```python
from build123d import *
from build123d.topology import SkipClean

# Parameters (mm, degrees)
CROQUIS1_R                          = 15
CROQUIS1_R_2                        = 10.5
SALIENTE_EXTRUIR1_DEPTH             = 4
CROQUIS2_R                          = 1.875
CORTAR_EXTRUIR1_DEPTH               = 8
SALIENTE_EXTRUIR2_REACH             = 35.779
SALIENTE_EXTRUIR2_END_RADIUS        = 15
CROQUIS2_4_R                        = 1.875
SALIENTE_EXTRUIR2_DIRECTION_2_DEPTH = 2
REVOLUCI_N1_ANGLE                   = 20
REVOLUCI_N1_OTHER_WAY_ANGLE         = 20
CORTAR_EXTRUIR6_DEPTH               = 35.481879299
CORTAR_EXTRUIR6_DEPTH_BACK          = 3
CROQUIS4_3_R                        = 1.875
CORTAR_EXTRUIR7_DEPTH               = 35.481879299
CORTAR_EXTRUIR8_START               = -8
CORTAR_EXTRUIR8_DEPTH               = 8
REDONDEO3_R                         = 1
SALIENTE_EXTRUIR3_START             = 5
SALIENTE_EXTRUIR3_DEPTH             = 5
CORTAR_EXTRUIR9_DEPTH               = 1.75
CORTAR_EXTRUIR9_DEPTH_BACK          = 0.5
SALIENTE_EXTRUIR4_OUTLINE_R         = 1.875
SALIENTE_EXTRUIR4_DEPTH             = 2.75
CORTAR_EXTRUIR10_DEPTH              = 3


# Read off the part's stored shape, not the designer's step: Cortar-Extruir8, Saliente-Extruir4
with BuildPart() as part:
    # Croquis1 → Saliente-Extruir1 (new, symmetric)
    with BuildSketch(Plane(origin=(0, 0, 0), x_dir=(1, 0, 0), z_dir=(0, 1, 0))):
        with Locations(Location((0, 0, 0), (0, 0, 270))):
            Circle(CROQUIS1_R)
        with Locations(Location((0, 0, 0), (0, 0, 270))):
            Circle(CROQUIS1_R_2, mode=Mode.SUBTRACT)
    extrude(amount=SALIENTE_EXTRUIR1_DEPTH, both=True)

    # Croquis2 → Cortar-Extruir1 (cut)
    with BuildSketch(Plane(origin=(0, 0, -15), x_dir=(-1, 0, 0), z_dir=(0, 0, -1))):
        Polygon((-3.2, 0), (-1.6, -2.771281292), (1.6, -2.771281292), (3.2, 0), (1.6, 2.771281292), (-1.6, 2.771281292), align=None)
        Circle(CROQUIS2_R)
    extrude(amount=-CORTAR_EXTRUIR1_DEPTH, mode=Mode.SUBTRACT)

    # Saliente-Extruir2: up to this cylinder (the profile starts outside it)
    with SkipClean():  # the faces are left unmerged after this step: merging them gives an invalid solid
        saliente_extruir2_end = Plane(origin=(0, -1.641104, 0), z_dir=(0, -1, 0)) * Cylinder(SALIENTE_EXTRUIR2_END_RADIUS, 103.15359, mode=Mode.PRIVATE)
        # Croquis2<4> → Saliente-Extruir2 (add, up to the surface)
        with BuildSketch(Plane(origin=(0, 0, -15), x_dir=(-1, 0, 0), z_dir=(0, 0, -1)), mode=Mode.PRIVATE) as saliente_extruir2_sk1:
            Polygon((-4.618802154, 0), (-2.309401077, -4), (2.309401077, -4), (4.618802154, 0), (2.309401077, 4), (-2.309401077, 4), align=None)
            Polygon((-1.6, -2.771281292), (1.6, -2.771281292), (3.2, 0), (1.6, 2.771281292), (-1.6, 2.771281292), (-3.2, 0), align=None, mode=Mode.SUBTRACT)
        saliente_extruir2_tool1 = extrude(saliente_extruir2_sk1.sketch, amount=-SALIENTE_EXTRUIR2_REACH, mode=Mode.PRIVATE) - saliente_extruir2_end
        add(saliente_extruir2_tool1.solids().sort_by_distance((3.358272, -1.938899, -15))[0])
        add(saliente_extruir2_tool1.solids().sort_by_distance((3.358272, -1.938899, -15))[1])
        # Croquis2<4> → Saliente-Extruir2 (add, up to the surface)
        with BuildSketch(Plane(origin=(0, 0, -15), x_dir=(-1, 0, 0), z_dir=(0, 0, -1)), mode=Mode.PRIVATE) as saliente_extruir2_sk2:
            Polygon((-3.2, 0), (-1.6, -2.771281292), (1.6, -2.771281292), (3.2, 0), (1.6, 2.771281292), (-1.6, 2.771281292), align=None)
            Circle(CROQUIS2_4_R, mode=Mode.SUBTRACT)
        saliente_extruir2_tool2 = extrude(saliente_extruir2_sk2.sketch, amount=-SALIENTE_EXTRUIR2_REACH, mode=Mode.PRIVATE) - saliente_extruir2_end
        add(saliente_extruir2_tool2.solids().sort_by_distance((2.326679, -1.343309, -15))[0])
        add(saliente_extruir2_tool2.solids().sort_by_distance((2.326679, -1.343309, -15))[1])

    # Croquis2<4> → Saliente-Extruir2 direction 2 (add)
    # profile 1 of 2: a face of its own
    with BuildSketch(Plane(origin=(0, 0, -15), x_dir=(-1, 0, 0), z_dir=(0, 0, -1))):
        Polygon((-4.618802154, 0), (-2.309401077, -4), (2.309401077, -4), (4.618802154, 0), (2.309401077, 4), (-2.309401077, 4), align=None)
        Polygon((-1.6, -2.771281292), (1.6, -2.771281292), (3.2, 0), (1.6, 2.771281292), (-1.6, 2.771281292), (-3.2, 0), align=None, mode=Mode.SUBTRACT)
    # profile 2 of 2: a face of its own
    with BuildSketch(Plane(origin=(0, 0, -15), x_dir=(-1, 0, 0), z_dir=(0, 0, -1))):
        Polygon((-3.2, 0), (-1.6, -2.771281292), (1.6, -2.771281292), (3.2, 0), (1.6, 2.771281292), (-1.6, 2.771281292), align=None)
        Circle(CROQUIS2_4_R, mode=Mode.SUBTRACT)
    extrude(amount=SALIENTE_EXTRUIR2_DIRECTION_2_DEPTH)

    # Croquis3 → Revolución1 (revolve)
    with BuildSketch(Plane(origin=(0, 0, 0), x_dir=(0, 0, -1), z_dir=(1, 0, 0))):
        Polygon((-30, 4), (-14, 4), (-14, -4), (-30, -4), (-30, -2.5), (-15, -2.5), (-15, 2.5), (-30, 2.5), align=None)
    revolve(axis=Axis((0, 4, 0), (0, -1, 0)), revolution_arc=REVOLUCI_N1_ANGLE)

    # Croquis3 → Revolución1 other way (revolve)
    with BuildSketch(Plane(origin=(0, 0, 0), x_dir=(0, 0, -1), z_dir=(1, 0, 0))):
        Polygon((-30, 4), (-14, 4), (-14, -4), (-30, -4), (-30, -2.5), (-15, -2.5), (-15, 2.5), (-30, 2.5), align=None)
    revolve(axis=Axis((0, 4, 0), (0, 1, 0)), revolution_arc=REVOLUCI_N1_OTHER_WAY_ANGLE)

    # Croquis4 → Cortar-Extruir6 (cut, two sides: drawn at the far end of the back side and taken through both)
    with BuildSketch(Plane.XZ.offset(4).offset(-CORTAR_EXTRUIR6_DEPTH_BACK)):
        with BuildLine():
            ThreePointArc((8.584705597, 23.586284782), (4.358569265, 24.7186746), (1.2e-08, 25.1))
            ThreePointArc((1.2e-08, 25.1), (-3.1, 22.000000006), (0, 18.9))
            ThreePointArc((0, 18.9), (3.281950558, 18.612866532), (6.464180709, 17.760190533))
            Line((6.464180709, 17.760190533), (8.584705597, 23.586284782))
        make_face()
    extrude(amount=CORTAR_EXTRUIR6_DEPTH + CORTAR_EXTRUIR6_DEPTH_BACK, mode=Mode.SUBTRACT)

    # Croquis4<3> → Cortar-Extruir7 (cut, through all)
    with BuildSketch(Plane.XZ.offset(4)):
        with Locations(Location((0, 22, 0), (0, 0, 270))):
            Circle(CROQUIS4_3_R)
    extrude(amount=-CORTAR_EXTRUIR7_DEPTH, mode=Mode.SUBTRACT)

    # Cortar-Extruir8 outline → Cortar-Extruir8 (cut)
    with BuildSketch(Plane.XZ.offset(4).offset(CORTAR_EXTRUIR8_START)):
        with BuildLine():
            ThreePointArc((-7.184552477, 19.7393957), (-6.262942497, 26.739718497), (1e-09, 30))
            ThreePointArc((1e-09, 30), (-5.20944533, 29.544232591), (-10.2606043, 28.190778624))
            Line((-10.2606043, 28.190778624), (-7.184552477, 19.7393957))
        make_face()
        with BuildLine():
            Line((7.184552477, 19.7393957), (8.584705598, 23.586284782))
            Line((8.584705598, 23.586284782), (10.2606043, 28.190778624))
            ThreePointArc((10.2606043, 28.190778624), (5.209445331, 29.54423259), (1e-09, 30))
            ThreePointArc((1e-09, 30), (6.262942498, 26.739718496), (7.184552477, 19.7393957))
        make_face()
    extrude(amount=CORTAR_EXTRUIR8_DEPTH, mode=Mode.SUBTRACT)

    # Redondeo3
    redondeo3_edges = [part.edges().sort_by_distance(p)[0] for p in [
        (6.464180709, -3.25, 17.760190533),
        (7.474898271, -3.25, 23.961133025),
        (-5.13030215, 3.25, 14.095389312),
        (-5.13030215, -3.25, 14.095389312),
        (5.13030215, 3.25, 14.095389312),
        (5.13030215, -3.25, 14.095389312),
    ]]
    fillet(redondeo3_edges, radius=REDONDEO3_R)

    # Croquis9 → Saliente-Extruir3 (add)
    with BuildSketch(Plane(origin=(0, -2.5, 0), x_dir=(1, 0, 0), z_dir=(0, 1, 0)).offset(SALIENTE_EXTRUIR3_START)):
        with BuildLine():
            Line((6.112599464, -16.794229002), (5.461623706, -15.005687805))
            ThreePointArc((5.461623706, -15.005687805), (5.482238333, -14.26959198), (6.001234056, -13.747188433))
            ThreePointArc((6.001234056, -13.747188433), (0, -15), (-6.001234056, -13.747188433))
            ThreePointArc((-6.001234056, -13.747188433), (-5.482238333, -14.26959198), (-5.461623706, -15.005687805))
            Line((-5.461623706, -15.005687805), (-7.184552477, -19.7393957))
            ThreePointArc((-7.184552477, -19.7393957), (-3.08103884, -29.351717504), (6.779967306, -25.888177056))
            ThreePointArc((6.779967306, -25.888177056), (6.683772805, -24.813619231), (5.667398999, -24.451801336))
            ThreePointArc((5.667398999, -24.451801336), (2.852173422, -24.93742382), (0, -25.1))
            ThreePointArc((0, -25.1), (-3.1, -22), (0, -18.9))
            ThreePointArc((0, -18.9), (2.760553354, -18.697308501), (5.461896053, -18.0935815))
            ThreePointArc((5.461896053, -18.0935815), (6.067051121, -17.584028122), (6.112599464, -16.794229002))
        make_face()
    extrude(amount=-SALIENTE_EXTRUIR3_DEPTH)

    # Croquis10 → Cortar-Extruir9 (cut, two sides: drawn at the far end of the back side and taken through both)
    with BuildSketch(Plane(origin=(0, -0.75, 0), x_dir=(-1, 0, 0), z_dir=(0, -1, 0)).offset(-CORTAR_EXTRUIR9_DEPTH_BACK)):
        with BuildLine():
            ThreePointArc((-6.779967306, -25.888177056), (-6.668671988, -26.09396334), (-6.551132513, -26.296248074))
            ThreePointArc((-6.551132513, -26.296248074), (-3.300127057, -26.898311497), (0, -27.1))
            ThreePointArc((0, -27.1), (5.1, -22), (0, -16.9))
            ThreePointArc((0, -16.9), (-1.942951583, -16.787940289), (-3.860136706, -16.453247236))
            ThreePointArc((-3.860136706, -16.453247236), (-4.828629021, -16.195503752), (-5.780140422, -15.880805291))
            Line((-5.780140422, -15.880805291), (-6.112599464, -16.794229002))
            ThreePointArc((-6.112599464, -16.794229002), (-6.067051121, -17.584028122), (-5.461896053, -18.0935815))
            ThreePointArc((-5.461896053, -18.0935815), (-2.760553354, -18.697308501), (0, -18.9))
            ThreePointArc((0, -18.9), (3.1, -22), (0, -25.1))
            ThreePointArc((0, -25.1), (-2.852173422, -24.93742382), (-5.667398999, -24.451801336))
            ThreePointArc((-5.667398999, -24.451801336), (-6.683772805, -24.813619231), (-6.779967306, -25.888177056))
        make_face()
    extrude(amount=CORTAR_EXTRUIR9_DEPTH + CORTAR_EXTRUIR9_DEPTH_BACK, mode=Mode.SUBTRACT)

    # Saliente-Extruir4 outline → Saliente-Extruir4 (add)
    with BuildSketch(Plane.XZ.offset(-2.5)):
        with BuildLine():
            ThreePointArc((5.461896053, 18.0935815), (6.067051121, 17.584028122), (6.112599464, 16.794229002))
            Line((6.112599464, 16.794229002), (7.184552477, 19.7393957))
            ThreePointArc((7.184552477, 19.7393957), (7.629143545, 22.856350834), (6.779967306, 25.888177056))
            ThreePointArc((6.779967306, 25.888177056), (6.683772805, 24.813619231), (5.667398999, 24.451801336))
            ThreePointArc((5.667398999, 24.451801336), (2.852173422, 24.93742382), (0, 25.1))
            ThreePointArc((0, 25.1), (-3.1, 22), (0, 18.9))
            ThreePointArc((0, 18.9), (2.760553354, 18.697308501), (5.461896053, 18.0935815))
        make_face()
        with Locations((0, 22)):
            Circle(SALIENTE_EXTRUIR4_OUTLINE_R, mode=Mode.SUBTRACT)
    extrude(amount=SALIENTE_EXTRUIR4_DEPTH)

    # Croquis12 → Cortar-Extruir10 (cut)
    with BuildSketch(Plane.XZ.offset(0.25)):
        Polygon((-2.771281292, 23.6), (-2.771281292, 20.4), (0, 18.8), (2.771281292, 20.4), (2.771281292, 23.6), (0, 25.2), align=None)
    extrude(amount=-CORTAR_EXTRUIR10_DEPTH, mode=Mode.SUBTRACT)


solid = part.part
```
Verification items for the finished model (mm, model axes). A direction names the side the tool comes from. Give positions to 0.01 mm unless a question says otherwise; leave off trailing zeros. Order: outer loops, then holes, each group sorted by start corner. A loop starts at its lowest first (then second) coordinate and runs counter-clockwise, first axis right, second up. Notation, with made-up numbers: (76, 63) -> (111, 63) arc R31 ccw to (111, 99) -> close; hole circle Ø9 at (-23, 69.25). An arc over 180 degrees is marked (long way). Use a Markdown table: item, result.
1) Section check C-C, the plane y = 0.5. Record the boundary of the cut face in (x, z), then the cut area to 3 significant figures.
Results:
| item | result |
|---|---|
| outline | (-7.18, 19.74) -> (-5.46, 15.01) arc R1 cw to (-6, 13.75) arc R15 ccw to (-4.33, -14.36) -> (-4.33, -17) -> (-1.81, -17) -> (-1.81, -14.89) arc R15 cw to (-2.91, -14.71) -> (-2.91, -10.09) arc R10.5 cw (long way) to (2.91, -10.09) -> (2.91, -14.71) arc R15 cw to (1.81, -14.89) -> (1.81, -17) -> (4.33, -17) -> (4.33, -14.36) arc R15 ccw to (6, 13.75) arc R1 cw to (5.46, 15.01) -> (7.18, 19.74) arc R7.65 ccw (long way) to start; hole (-2.77, 20.4) -> (0, 18.8) -> (2.77, 20.4) -> (2.77, 23.6) -> (0, 25.2) -> (-2.77, 23.6) -> close |
| area | 514 mm² |
2) Tool access check on faces 4 (the cylindrical face through (-3.1, -3.2, 22.1)), 5 (the flat face through (3.48, -1.97, -15.62)), 6 (the flat face through (3.448, 2.028, -15.92)), 7 (the cylindrical face through (6.072, -3.26, 17.574)), 8 (the flat face through (2.41, -1.37, -12.49)). Record the directions out of +Z, -Z, +X, -X, +Y, -Y that give a thin tool (end or side, any length) a straight path to the whole face; none if there is none.
Results:
| item | result |
|---|---|
| face 4 | -Y |
| face 5 | -Z, +X, -Y |
| face 6 | -Z, +X, +Y |
| face 7 | +X, -Y |
| face 8 | none |
3) Section check A-A, the plane z = 0. Record the boundary of the cut face in (x, y), then the cut area to 3 significant figures.
Results:
| item | result |
|---|---|
| outline | (-15, -4) -> (-10.5, -4) -> (-10.5, 4) -> (-15, 4) -> close; (10.5, -4) -> (15, -4) -> (15, 4) -> (10.5, 4) -> close |
| area | 72.0 mm² |
4) Depth check by flat-ended pin: pin 1 Ø2.5 at (y, z) = (1, 21.5) entering from -X; pin 2 Ø4 at (y, z) = (-1, 14) entering from +X; pin 3 Ø4.5 at (x, z) = (0, 22) entering from -Y; pin 4 Ø5.5 at (x, z) = (0, 23) entering from -Y. Enter the tip coordinate at first touch or a pass-through.
Results:
| item | result |
|---|---|
| pin 1 | x = -7.65 |
| pin 2 | x = 9 |
| pin 3 | y = 2.75 |
| pin 4 | y = -4 |
5) Material ranges on probe 1 along X at (y, z) = (1, 0); probe 2 along Z at (x, y) = (-2.5, -1.75); probe 3 along X at (y, z) = (3.2, 22) (3 decimals), recorded low to high.
Results:
| item | result |
|---|---|
| probe 1 | -15 to -10.5, 10.5 to 15 |
| probe 2 | -17 to -10.2, 10.2 to 17.55, 26.45 to 29.58 |
| probe 3 | -7.637 to -1.875, 1.875 to 7.637 |
6) Section check D-D, the plane z = 22. Record the boundary of the cut face in (x, y) (3 decimals), then the cut area to 3 significant figures.
Results:
| item | result |
|---|---|
| outline | (-7.637, -4) -> (-3.1, -4) -> (-3.1, -2.5) -> (-5.1, -2.5) -> (-5.1, -0.25) -> (-2.771, -0.25) -> (-2.771, 2.75) -> (-1.875, 2.75) -> (-1.875, 4) -> (-7.637, 4) -> close; (1.875, 2.75) -> (2.771, 2.75) -> (2.771, -0.25) -> (7.637, -0.25) -> (7.637, 4) -> (1.875, 4) -> close |
| area | 56.1 mm² |
7) Mould release check, pull along X, two halves, no side actions. Record for faces 1 (the cylindrical face through (14.91, 0.06, -1.65)), 2 (the flat face through (-3.48, 1.97, -15.62)), 3 (the flat face through (2.771, 1, 22)): pulls with the +X half, pulls with the -X half, needs draft (parallel to the pull), parting line crosses it, or undercut.
Results:
| item | result |
|---|---|
| face 1 | pulls with the +X half |
| face 2 | pulls with the -X half |
| face 3 | undercut |
8) Section check B-B, the plane x = -4. Record the boundary of the cut face in (y, z), then the cut area to 3 significant figures.
Results:
| item | result |
|---|---|
| outline | (-4, -14.46) -> (-1.07, -14.46) -> (-1.07, -17) -> (1.07, -17) -> (1.07, -14.46) -> (4, -14.46) -> (4, -9.71) -> (-4, -9.71) -> close; (-4, 9.71) -> (4, 9.71) -> (4, 28.87) -> (-4, 28.87) -> close; hole (-2.5, 18.84) -> (-0.25, 18.84) -> (-0.25, 25.16) -> (-2.5, 25.16) -> close |
| area | 182 mm² |
